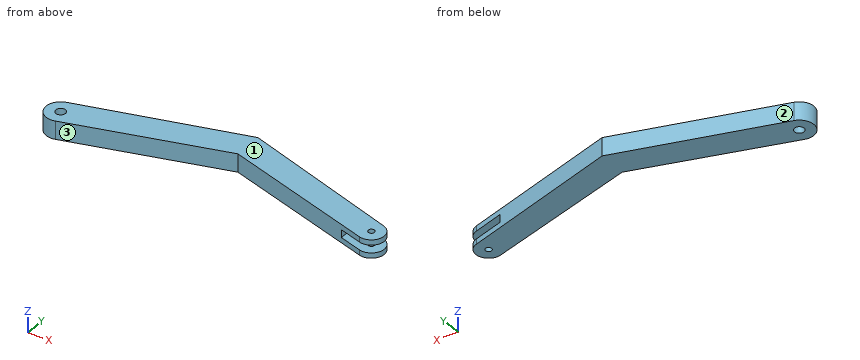
```python
from build123d import *

# Parameters (mm, degrees)
SKETCH1_R               = 0.79375
BOSS_EXTRUDE1_DEPTH     = 2.9718
SKETCH2_W               = 8.538559206
SKETCH2_H               = 1.27
CUT_EXTRUDE1_DEPTH      = 10.919149519
CUT_EXTRUDE1_DEPTH_BACK = 3.38125
SKETCH1_4_R             = 0.508
CUT_EXTRUDE3_DEPTH      = 3.9718
CUT_EXTRUDE3_DEPTH_BACK = 1


with BuildPart() as part:
    # Sketch1 → Boss-Extrude1 (new body)
    with BuildSketch(Plane.XY):
        with BuildLine():
            Line((-50.113827643, -2.280245394), (-25.4, 5.156649519))
            Line((-25.4, 5.156649519), (-0.581588952, -2.013175239))
            ThreePointArc((-0.581588952, -2.013175239), (2.009011043, -0.595814467), (0.610010171, 2.004746329))
            Line((0.610010171, 2.004746329), (-25.4, 9.919149519))
            Line((-25.4, 9.919149519), (-51.469201485, 2.285283557))
            ThreePointArc((-51.469201485, 2.285283557), (-53.082780246, -0.677691603), (-50.113827643, -2.280245394))
        make_face()
        with Locations((-50.8, 0)):
            Circle(SKETCH1_R, mode=Mode.SUBTRACT)
    extrude(amount=BOSS_EXTRUDE1_DEPTH)

    # Sketch2 → Cut-Extrude1 (cut, two sides)
    with BuildSketch(Plane(origin=(0, 0, 0), x_dir=(1, 0, 0), z_dir=(0, 1, 0))) as cut_extrude1_sk:
        with Locations((0.014779603, -1.4859)):
            Rectangle(SKETCH2_W, SKETCH2_H)
    extrude(amount=CUT_EXTRUDE1_DEPTH, mode=Mode.SUBTRACT)
    extrude(cut_extrude1_sk.sketch, amount=-CUT_EXTRUDE1_DEPTH_BACK, mode=Mode.SUBTRACT)

    # Sketch1<4> → Cut-Extrude3 (cut, two sides)
    with BuildSketch(Plane.XY) as cut_extrude3_sk:
        Circle(SKETCH1_4_R)
    extrude(amount=CUT_EXTRUDE3_DEPTH, mode=Mode.SUBTRACT)
    extrude(cut_extrude3_sk.sketch, amount=-CUT_EXTRUDE3_DEPTH_BACK, mode=Mode.SUBTRACT)


solid = part.part
```
Here's how the part is built. I have some questions about the finished solid (model axes, mm). Face numbers are marked on the shaded views. Give positions to 0.01 mm unless a question says otherwise; leave off trailing zeros. Order: outer loops, then holes, each group sorted by start corner. A loop starts at its lowest first (then second) coordinate and runs counter-clockwise, first axis right, second up. Notation, with made-up numbers: (0.5, 4) - (59.5, 4) arc R12 cw to (59.5, 21) - close; hole circle Ø4 at (0.5, 14). An arc over 180 degrees is marked (long way). Answer as a JSON object with one key per item and string values. Group by question number.
Item 1: If we section it at B-B on z = 1.3: Please give me the cut outline in (x, y).
Item 2: If we section it at D-D on y = 0: Please give me the cut outline in (x, z), and give its area (3 significant figures).
Item 3: If we mould it in two halves opening along X, with no side actions, what happens to the marked faces 1, 2 and 3? For each: pulls with the +X half, pulls with the -X half, needs draft (parallel to the pull), parting line crosses it, or undercut.
Item 4: If we section it at A-A on y = 4.5: Please give me the cut outline in (x, z), and give its area (3 significant figures).
Item 5: Please list where these lines run through material, in increasing order: probe 1 along Y at (x, z) = (-50.8, 1.6); probe 2 along Y at (x, z) = (0, 2.8); probe 3 along Y at (x, z) = (-12.5, 0.8).
Item 6: For P1, Ø0.6, axis at x = 0, y = 0, coming from the +Z side (3 decimals); P2, Ø0.6, axis at y = 1.5, z = 1.5, coming from the +X side; P3, Ø1, axis at y = 1.5, z = 0.5, coming from the -X side, each with a flat end and sliding along its axis, tell me the tip position at first contact or that it passes through.
Item 7: If we section it at C-C on x = -50.8: Please give me the cut outline in (y, z).
Result set:
{
 "1": {"outline": "(-51.47, 2.29) arc R2.38 ccw (long way) to (-50.11, -2.28) - (-25.4, 5.16) - (-4.25, -0.95) - (-4.25, 3.48) - (-25.4, 9.92) - close; hole circle Ø1.59 at (-50.8, 0)"},
 "2": {"outline": "(-53.18, 0) - (-51.59, 0) - (-51.59, 2.97) - (-53.18, 2.97) - close; (-50.01, 0) - (-42.54, 0) - (-42.54, 2.97) - (-50.01, 2.97) - close; (-7.55, 0) - (-0.51, 0) - (-0.51, 0.85) - (-4.25, 0.85) - (-4.25, 2.12) - (-0.51, 2.12) - (-0.51, 2.97) - (-7.55, 2.97) - close; (0.51, 0) - (2.1, 0) - (2.1, 0.85) - (0.51, 0.85) - close; (0.51, 2.12) - (2.1, 2.12) - (2.1, 2.97) - (0.51, 2.97) - close", "area": "45.8 mm²"},
 "3": {"face 1": "needs draft", "face 2": "pulls with the -X half", "face 3": "undercut"},
 "4": {"outline": "(-43.91, 0) - (-27.58, 0) - (-27.58, 2.97) - (-43.91, 2.97) - close; (-23.13, 0) - (-7.59, 0) - (-7.59, 2.97) - (-23.13, 2.97) - close", "area": "94.7 mm²"},
 "5": {"probe 1": "-2.38 to -0.79, 0.79 to 2.48", "probe 2": "-2.1 to -0.51, 0.51 to 2.19", "probe 3": "1.43 to 5.99"},
 "6": {"P1": "through", "P2": "x = -4.25", "P3": "x = -52.96"},
 "7": {"outline": "(-2.38, 0) - (-0.79, 0) - (-0.79, 2.97) - (-2.38, 2.97) - close; (0.79, 0) - (2.48, 0) - (2.48, 2.97) - (0.79, 2.97) - close"}
}
